Source: three-view drawing plus pictorial views. Frame: mm from the lowest corner of the part. Give positions to 0.01 mm unless a question says otherwise; leave off trailing zeros. Write each loop counter-clockwise with the first axis right and the second up, starting at its lowest first coordinate (ties: lowest second). Pieces come first, ordered by that corner, then holes.
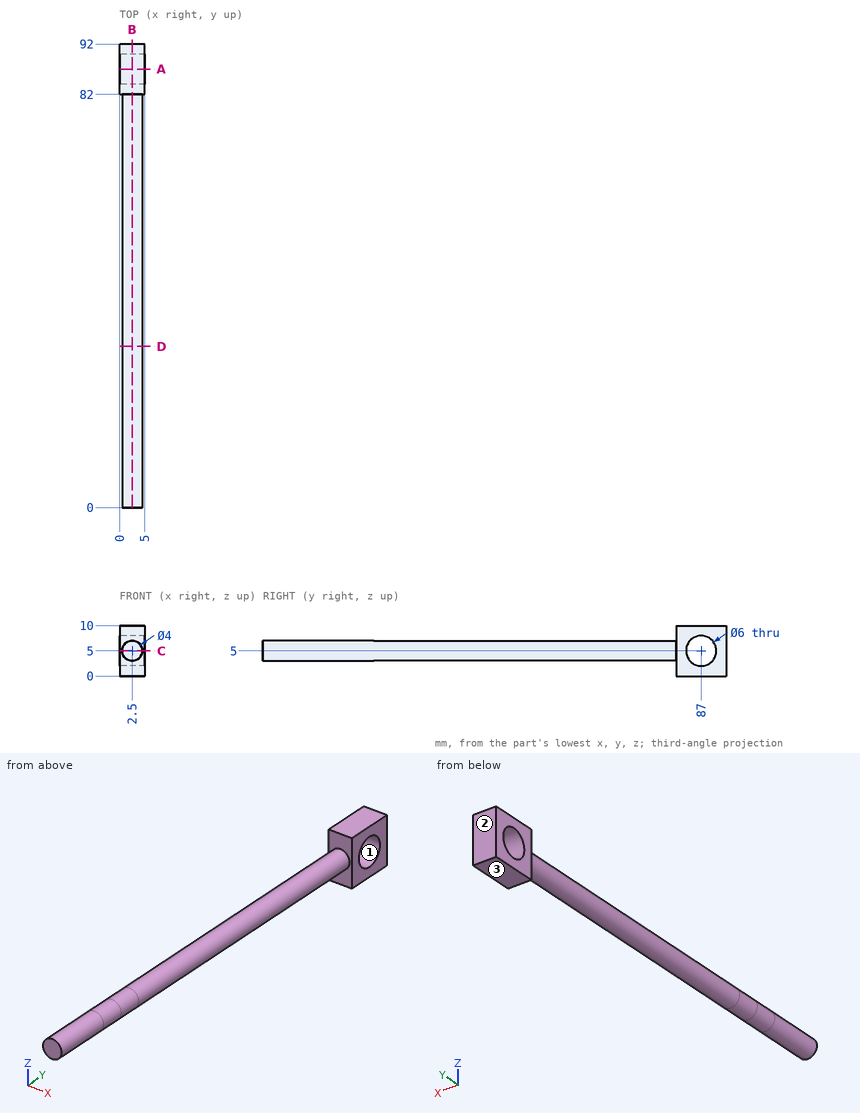
Q1. Section D-D on y = 32. Output: boundary loops of the cut face in (x, z), plus the area to 3 significant figures.
Filled sheet:
outline: circle Ø4 at (2.5, 5)
area: 12.6 mm2
Q2. Pin query (flat end, axial travel): P1, Ø1.5, axis at y = 60.5, z = 2, coming from the +X side; P2, Ø6, axis at y = 31, z = 1.5, coming from the +X side; P3, Ø3, axis at x = 4, y = 43, coming from the +Z side; P4, Ø1.5, axis at y = 38, z = 4, coming from the -X side. Return the tip coordinate at first contact, or that it passes through.
Filled sheet:
P1: passes through
P2: stops at x = 4.44
P3: stops at z = 7
P4: stops at x = 0.52
Q3. Pull-direction query (Z, two-part tool) for the marked faces 1, 2 and 3; classes: released by +Z, released by -Z, zero draft, split by the parting line, or undercut.
Filled sheet:
face 1: undercut
face 2: zero draft
face 3: released by -Z
Q4. Section B-B on x = 2.5. Output: boundary loops of the cut face in (y, z), plus the area to 3 significant figures.
Filled sheet:
outline: (0, 3) - (82, 3) - (82, 0) - (92, 0) - (92, 10) - (82, 10) - (82, 7) - (0, 7) - close; hole circle Ø6 at (87, 5)
area: 400 mm2
Q5. Section C-C on z = 5. Output: boundary loops of the cut face in (x, y), plus the area to 3 significant figures.
Filled sheet:
outline: (0, 82) - (0.5, 82) - (0.5, 0) - (4.5, 0) - (4.5, 82) - (5, 82) - (5, 84) - (0, 84) - close; (0, 90) - (5, 90) - (5, 92) - (0, 92) - close
area: 348 mm2
Q6. Section A-A on y = 87. Output: boundary loops of the cut face in (x, z), plus the area to 3 significant figures.
Filled sheet:
outline: (0, 0) - (5, 0) - (5, 2) - (0, 2) - close; (0, 8) - (5, 8) - (5, 10) - (0, 10) - close
area: 20.0 mm2
Q7. Ray query, line 1 along Y through (x, z) = (1.3, 5); line 2 along Y through (x, z) = (1.6, 7.5); line 3 along X through (y, z) = (41, 5.25). Return the intervals inside material, ascending.
Filled sheet:
line 1: y = 0 to 84, 90 to 92
line 2: y = 82 to 85.34, 88.66 to 92
line 3: x = 0.52 to 4.48
